Read the model definition and answer for the solid it produces. Units are mm, in the model's axes. Face numbers are marked on the shaded views. A direction names the side the tool comes from. Give positions to 0.01 mm unless a question says otherwise; leave off trailing zeros. Write each loop counter-clockwise with the first axis right and the second up, starting at its lowest first coordinate (ties: lowest second). Pieces come first, ordered by that corner, then holes. Notation, with made-up numbers: (61.5, -36) -> (67.5, -36) arc R7 ccw to (67.5, -24) -> close; hole circle Ø1 at (76, 31). An arc over 180 degrees is marked (long way). Put each result on its own line as item: value. Start each with the question number.
Autodesk Inventor part; units mm, degrees
ref_plane "YZ Plane" through (0, 0, 0) normal (1, 0, 0) x (0, 1, 0)
ref_plane "XZ Plane" through (0, 0, 0) normal (0, 1, 0) x (-1, 0, 0)
ref_plane "XY Plane" through (0, 0, 0) normal (0, 0, 1) x (1, 0, 0)
sketch "Sketch1" plane through (0, 0, 0) normal (1, 0, 0) x (0, 1, 0)
  line L0 (0, 0) -> (7.5, 0)
  line L1 (7.5, 0) -> (7.5, -12.5)
  line L2 (7.5, -12.5) -> (0, -12.5)
  line L3 (0, -12.5) -> (0, 0)
  circle A0 centre (2.5, -2.5) radius 1.5
  circle A1 centre (2.5, -10) radius 1.5
  line L4 (2.5, -2.5) -> (2.5, -10) construction
  line L5 (7.5, -12.5) -> (7.5, 0)
  point P0 (2.5, -6.25)
  point P1 (7.5, -6.25)
  point P2 (3.75, -12.5)
  dimension "d0" = 12.5
  dimension "d1" = 7.5
  dimension "d2" = 3
  dimension "d3" = 7.5
  dimension "d4" = 5
extrude "Extrusion1" add sketch "Sketch1" along normal blind 5
sketch "Sketch2" plane through (5, 0, 0) normal (1, 0, 0) x (0, 0, -1)
  line L0 (12.5, 7.5) -> (0, 7.5)
  line L1 (0, 7.5) -> (0, 0)
  line L2 (0, 7.5) -> (0, 52.5)
  line L3 (0, 52.5) -> (10, 52.5)
  line L4 (10, 52.5) -> (10, 7.5)
  dimension "d7" = 10
  dimension "d8" = 45
extrude "Extrusion2" add sketch "Sketch2" against normal blind 5
sketch "Sketch3" plane through (5, 7.5, -10) normal (0, 0, -1) x (-1, 0, 0)
  circle A0 centre (5, 53.6603) radius 10
  circle A1 centre (5, 53.6603) radius 6
  line L0 (0, 45) -> (5, 45)
  point P0 (5, -7.5)
  point P1 (2.5, 45)
  dimension "d11" = 12
  dimension "d12" = 4
extrude "Extrusion3" add sketch "Sketch3" against normal up to surface (10 mm away)
fillet "Fillet1" radius 5 3 edges at (5, 52.5, -5) (0, 51.1603, -5) (2.5, 7.5, -10)
properties part number "LJ12_Adapter"
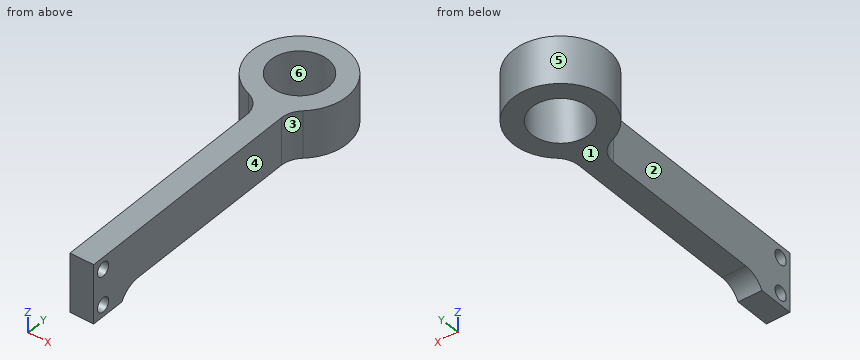
1) For a pull along Y with two mould halves and no side action, classify the marked faces 4, 5 and 6 as pulls with the +Y half, pulls with the -Y half, needs draft (parallel to the pull), parting line crosses it, or undercut.
2) For the marked faces 1, 2 and 3, determine the directions among +Z, -Z, +X, -X, +Y, -Y from which every point of the face is accessible in a straight line to the end or side of a thin tool.
3) A cutting plane is placed at A-A on z = -2.5. Give the vertices of the cut face in (x, y).
4) A cutting plane is placed at D-D on x = -5.25. Give the vertices of the cut face in (y, z).
5) A cutting plane is placed at C-C on x = 1.5. Give the vertices of the cut face in (y, z).
6) Each of these flat-tipped pins is pushed along its axis until it touches: pin 1 Ø8 at (x, y) = (0.5, 59.5) entering from -Z; pin 2 Ø1 at (x, z) = (-5.5, -4) entering from +Y; pin 3 Ø3.5 at (y, z) = (2.5, -2.5) entering from -X; pin 4 Ø2 at (y, z) = (54, -7.5) entering from -X. Where does it stop, or does it pass through?
7) Straight lines are drawn through the part: line 1 (Z direction, x = 3.1, y = 2.5); line 2 (Z direction, x = 8.75, y = 64.5); line 3 (X direction, y = 60.5, z = -0.75). For each, find the intervals that lie inside material, in ascending order. Write a range as [from, to].
8) A cutting plane is placed at B-B on y = 2.5. Give the vertices of the cut face in (x, z), and give its area (3 significant figures).
Results found:
1. face 4: needs draft
1. face 5: parting line crosses it
1. face 6: undercut
2. face 1: -Z, +X, -X, +Y
2. face 2: +Z, -Z, -X, -Y
2. face 3: +Z, -Z, +X, -Y
3. outline: (-3.33, 51.73) arc R5 cw to (0, 47.02) -> (0, 4) -> (5, 4) -> (5, 49.98) arc R5 cw to (6.67, 53.71) arc R10 ccw (long way) to start; (0, 0) -> (5, 0) -> (5, 1) -> (0, 1) -> close; hole circle Ø12 at (0, 61.16)
4. outline: (52.65, -10) -> (58.26, -10) -> (58.26, 0) -> (52.65, 0) -> close; (64.07, -10) -> (69.67, -10) -> (69.67, 0) -> (64.07, 0) -> close
5. outline: (0, -12.5) -> (7.5, -12.5) arc R5 cw to (11.83, -10) -> (55.35, -10) -> (55.35, 0) -> (0, 0) -> close; (66.97, -10) -> (71.05, -10) -> (71.05, 0) -> (66.97, 0) -> close; hole circle Ø3 at (2.5, -10); hole circle Ø3 at (2.5, -2.5)
6. pin 1: passes through
6. pin 2: stops at y = 69.82
6. pin 3: stops at x = 0
6. pin 4: stops at x = -7.88
7. line 1: z = [-12.5, -11.5], [-8.5, -4], [-1, 0]
7. line 2: z = [-10, 0]
7. line 3: x = [-9.98, -5.96], [5.96, 9.98]
8. outline: (0, -12.5) -> (5, -12.5) -> (5, -11.5) -> (0, -11.5) -> close; (0, -8.5) -> (5, -8.5) -> (5, -4) -> (0, -4) -> close; (0, -1) -> (5, -1) -> (5, 0) -> (0, 0) -> close
8. area: 32.5 mm²
